Answer from the drawing. Dimensions are ordinates in mm from the lowest x, y and z of the part. A direction names the side the tool comes from. Coordinates: 2 decimals unless noted, no trailing zeros. Loops run counter-clockwise (first coordinate to the right, second up) from the corner with the lowest first, then second, coordinate; pieces in that order, holes last. Notation, with made-up numbers: (-7.75, 68.25) - (50.25, 68.25) arc R24 ccw to (50.25, 103.25) - close; hole circle Ø6 at (-25.75, 8.25). An arc over 180 degrees is marked (long way). Use one line per item in the form item = value. Start each with the question number.
1) Each of these flat-tipped pins is pushed along its axis until it touches: P1, Ø6, axis at x = 39.5, y = 56.5, coming from the +Z side; P2, Ø12, axis at x = 14, z = 47, coming from the +Y side; P3, Ø1.5, axis at x = 34.5, z = 28.5, coming from the -Y side. Where does it stop, or does it pass through?
2) A cutting plane is placed at B-B (z = 38.5). Give the vertices of the cut face in (x, y), and give its area (4 significant figures).
3) Consider line 1 (Z direction, x = 4, y = 12); line 2 (Y direction, x = 6, z = 55); line 3 (Z direction, x = 36.5, y = 93). Determine where each line is inside the solid, lowest interval first.
4) A cutting plane is placed at A-A (x = 25). Give the vertices of the cut face in (y, z).
5) A cutting plane is placed at D-D (y = 37.5). Give the vertices of the cut face in (x, z), and give its area (3 significant figures).
6) Which of the six approach directions +Z, -Z, +X, -X, +Y, -Y give full straight-line access (tool end or side, diameter ignored) to the marked faces 1, 2 and 3?
7) A cutting plane is placed at C-C (z = 8). Give the vertices of the cut face in (x, y).
8) The mould has two halves that part along X. Classify the marked faces 4, 5, 6 and 7: released by +X, released by -X, zero draft, split by the parting line, or undercut.
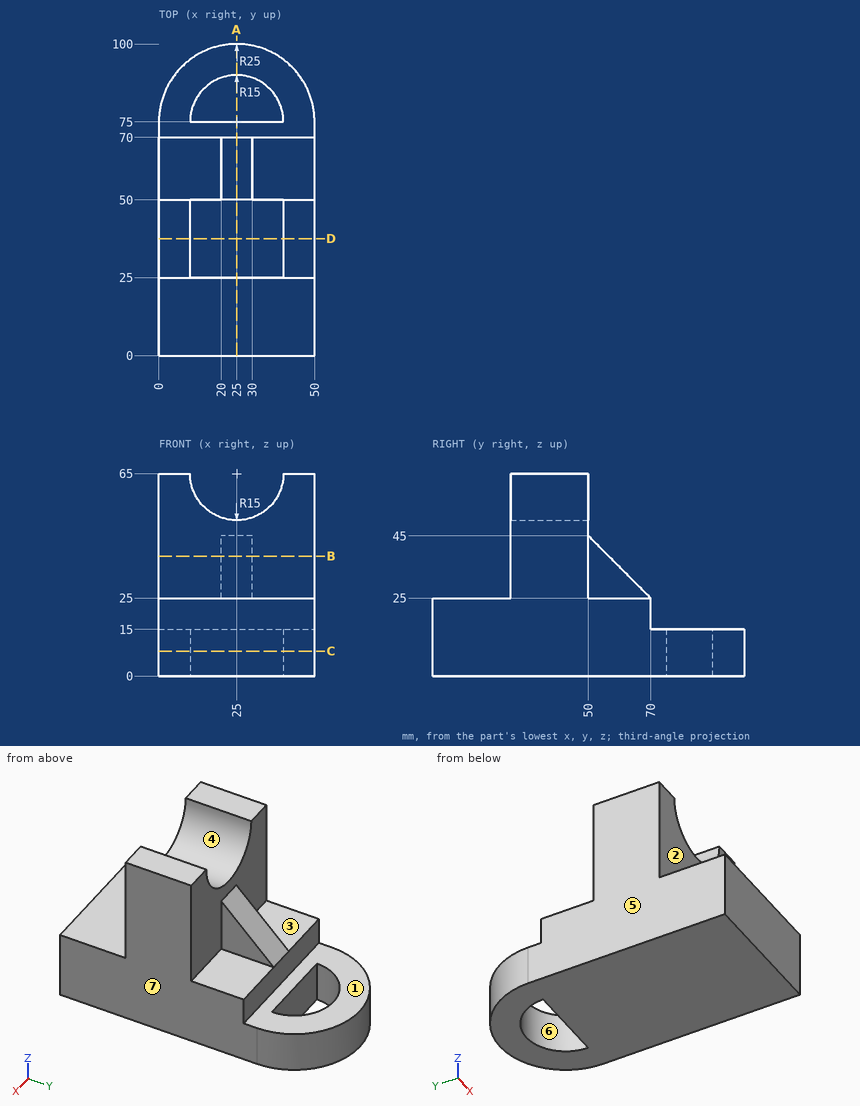
Found:
q1.P1 = 25
q1.P2 = 50
q1.P3 = 25
q2.outline = (0, 25) - (50, 25) - (50, 50) - (30, 50) - (30, 56.5) - (20, 56.5) - (20, 50) - (0, 50) - close
q2.area = 1,315 mm^2
q3.line_1 = 0 to 25
q3.line_2 = 25 to 50
q3.line_3 = 0 to 15
q4.outline = (0, 0) - (75, 0) - (75, 15) - (70, 15) - (70, 25) - (50, 45) - (50, 50) - (25, 50) - (25, 25) - (0, 25) - close; (90, 0) - (100, 0) - (100, 15) - (90, 15) - close
q5.outline = (0, 0) - (50, 0) - (50, 65) - (40, 65) arc R15 cw to (10, 65) - (0, 65) - close
q5.area = 2,900 mm^2
q6.face_1 = +Z, +X, -X, +Y
q6.face_2 = +Z, +X, -X, -Y
q6.face_3 = +Z, -X, +Y
q7.outline = (0, 0) - (50, 0) - (50, 75) arc R25 ccw to (0, 75) - close; hole (10, 75) - (40, 75) arc R15 ccw to start
q8.face_4 = undercut
q8.face_5 = released by -X
q8.face_6 = undercut
q8.face_7 = released by +X
